```python
from build123d import *

# Parameters (mm, degrees)
F0_R        = 22.3974192725
F1_DEPTH    = 30
F2_W        = 85
F2_H        = 50
F3_DEPTH    = 70
F4_W        = 38
F4_H        = 60.7357084751
F5_DEPTH    = 50
F6_T1_DEPTH = 50
F8_DEPTH    = 47
F9_R        = 11.0426148683
F10_DEPTH   = 47


# Not quite as in the source:
# - a fillet or chamfer that OpenCascade refuses, or shapes differently, is made with other operations: its cross-section is extruded or revolved along the edge and cut away or added


with BuildPart() as f1:
    # F0 (on Top) → F1 (new body)
    with BuildSketch(Plane.XY):
        with BuildLine():
            Line((0, 0), (0, 45))
            Line((0, 45), (-160, 45))
            ThreePointArc((-160, 45), (-205, 0), (-160, -45))
            Line((-160, -45), (0, -45))
            Line((0, -45), (0, 0))
        make_face()
        with Locations((-160, 0)):
            Circle(F0_R, mode=Mode.SUBTRACT)
    extrude(amount=F1_DEPTH)

    # F2 (on face) → F3 (join)
    with BuildSketch(Plane.XY.offset(30)):
        with Locations((-42.5, 0)):
            Rectangle(F2_W, F2_H)
    extrude(amount=F3_DEPTH)

    # F4 (on face) → F5 (cut)
    with BuildSketch(Plane.XZ.offset(25)):
        with Locations((-19, 69.6321457624)):
            Rectangle(F4_W, F4_H)
    extrude(amount=-F5_DEPTH, mode=Mode.SUBTRACT)

    # F6: fillet of radius 45.3872149726 on 1 edges, made by hand

    # F6_s2 → F6_t1 (join)
    with BuildSketch(Plane.XZ.offset(-25)):
        with BuildLine():
            ThreePointArc((0, 39.2642915249), (-27.2197525121, 54.6803835575), (-38, 84.0463006125))
            Line((-38, 84.0463006125), (-38, 39.2642915249))
            Line((-38, 39.2642915249), (0, 39.2642915249))
        make_face()
    extrude(amount=F6_T1_DEPTH)

    # F7 (on face) → F8 (join)
    with BuildSketch(Plane(origin=(-85, 0, 0), x_dir=(0, -1, 0), z_dir=(-1, 0, 0))):
        with BuildLine():
            Line((-25, 100), (25, 100))
            ThreePointArc((25, 100), (0, 125), (-25, 100))
        make_face()
    extrude(amount=-F8_DEPTH)

    # F9 (on face) → F10 (cut)
    with BuildSketch(Plane(origin=(-85, 0, 0), x_dir=(0, -1, 0), z_dir=(-1, 0, 0))):
        with Locations((0, 100)):
            Circle(F9_R)
    extrude(amount=-F10_DEPTH, mode=Mode.SUBTRACT)

    # F11: F1 across face


with BuildPart() as f1_1:
    add(f1.part)
    add(f1.part.mirror(Plane(origin=(0, 0, 17.8748906724), x_dir=(0, 1, 0), z_dir=(1, 0, 0))))


solid = f1_1.part
```
Source: CAD feature listing. Evaluate the final solid. Frame: model axes, mm. A direction names the side the tool comes from. Give positions to 0.01 mm unless a question says otherwise; leave off trailing zeros. Order: outer loops, then holes, each group sorted by start corner. A loop starts at its lowest first (then second) coordinate and runs counter-clockwise, first axis right, second up.
(1) Pull-direction query (X, two-part tool) for faces 6 (the face through (26.93, 0.35, 54.34)), 7 (the face through (3, -29, 30)), 8 (the face through (85, 0, 78)); classes: +X half, -X half, draft (parallel to the pull), parting line (faces both ways), or undercut.
(2) Access query for faces 1 (the face through (2, -45, 15)), 2 (the face through (-26.93, 0.35, 54.34)), 3 (the face through (204.99, 0.99, 14.79)), 4 (the face through (20, -25, 42)), 5 (the face through (-85, 0, 78)). Directions: +Z, -Z, +X, -X, +Y, -Y. A direction counts if a zero-diameter tool reaches every point of the face in a straight line with its end or side. Return the directions, or none.
(3) Section query C-C (x = -78). Return the cut outline in (y, z), plus the area to 3 significant figures.
(4) Section query B-B (z = 58.5). Return the cut outline in (x, y), plus the area to 3 significant figures.
(5) Section query A-A (y = 0). State how many separate pieces and enclosed holes the cut face has, plus the area to 3 significant figures.
(6) Section query D-D (z = 17). Return the cut outline in (x, y).
(7) Contact query for flat-ended pins moving along their axis: P1, Ø8, axis at y = -8.5, z = 15, coming from the -X side; P2, Ø8, axis at y = -6, z = 30.5, coming from the -X side; P3, Ø1.5, axis at x = 107.5, y = 10, coming from the -Z side; P4, Ø21, axis at x = 38, z = 74.5, coming from the -Y side. Output: stop coordinate, or through.
(8) Material intervals for line 1 along Y through (x, z) = (-160, 17.25); line 2 along X through (y, z) = (23, 95); line 3 along Z through (x, y) = (142, -31.5), sorted ascending.
Outcome:
1. face 6: undercut
1. face 7: draft
1. face 8: +X half
2. face 1: +Z, -Z, +X, -X, -Y
2. face 2: +Z, +Y, -Y
2. face 3: +Z, -Z, +X
2. face 4: +Z, +X, -X, -Y
2. face 5: +Z, -X, +Y, -Y
3. outline: (-45, 0) - (45, 0) - (45, 30) - (25, 30) - (25, 100) arc R25 ccw to (-25, 100) - (-25, 30) - (-45, 30) - close; hole circle Ø22.09 at (0, 100)
3. area: 6,800 mm2
4. outline: (-85, -25) - (-30.13, -25) - (-30.13, 25) - (-85, 25) - close; (30.13, -25) - (85, -25) - (85, 25) - (30.13, 25) - close
4. area: 5,490 mm2
5. separate pieces: 5
5. enclosed holes: 0
5. area: 18,000 mm2
6. outline: (-160, -45) - (160, -45) arc R45 ccw to (160, 45) - (-160, 45) arc R45 ccw to start; hole circle Ø44.79 at (-160, 0); hole circle Ø44.79 at (160, 0)
7. P1: stops at x = -204.77
7. P2: stops at x = -204.95
7. P3: stops at z = 0
7. P4: stops at y = -25
8. line 1: y = -45 to -22.4, 22.4 to 45
8. line 2: x = -85 to -38, 38 to 85
8. line 3: z = 0 to 30
